Verification items for the finished model (mm, model axes). A direction names the side the tool comes from. Coordinates: 2 decimals unless noted, no trailing zeros. Write each loop counter-clockwise with the first axis right and the second up, starting at its lowest first coordinate (ties: lowest second). Pieces come first, ordered by that corner, then holes. Notation, with made-up numbers: (-36, 84) -> (17, 84) arc R12 cw to (17, 98) -> close; hole circle Ø1 at (84.5, -32.5). An arc over 180 degrees is marked (long way). Use CSV: the item, a comma, the result in double quotes.
```python
from build123d import *

# Parameters (mm, degrees)
CHAMFER1_SIZE  = 1
CHAMFER1_SIZE2 = 0.267949192


with BuildPart() as part:
    # Sketch1 → Revolve1 (revolve)
    with BuildSketch(Plane(origin=(0, 0, 0), x_dir=(1, 0, 0), z_dir=(0, 1, 0))):
        Polygon((16, 0), (16, 10), (15, 10), (15, 20), (45, 20), (45, 10), (21, 10), (21, 0), align=None)
    revolve(axis=Axis((0, 0, 0), (0, 0, 1)))

    # Chamfer1
    chamfer1_edges = [part.edges().sort_by_distance(p)[0] for p in [
        (-16, 0, 0),
    ]]
    chamfer1_side = [part.faces().sort_by_distance(p)[0] for p in [
        (-16, 0, -5),
    ]]
    chamfer(chamfer1_edges, length=CHAMFER1_SIZE, length2=CHAMFER1_SIZE2, reference=chamfer1_side[0])


solid = part.part
```
1) Cross-section at A-A (x = 0). Record the boundary of the cut face in (y, z).
Return value:
outline,"(-45, -20) -> (-15, -20) -> (-15, -10) -> (-16, -10) -> (-16, -1) -> (-16.27, 0) -> (-21, 0) -> (-21, -10) -> (-45, -10) -> close; (15, -20) -> (45, -20) -> (45, -10) -> (21, -10) -> (21, 0) -> (16.27, 0) -> (16, -1) -> (16, -10) -> (15, -10) -> close"
2) Mould release check, pull along X, two halves, no side actions. Record for faces 3 (the flat face through (6.1, -15.5, 0)), 4 (the cylindrical face through (20.765, -39.923, -14.93)), 5 (the cylindrical face through (-3.47, -15.62, -5.56)): released by +X, released by -X, zero draft, split by the parting line, or undercut.
Return value:
face 3,"zero draft"
face 4,"split by the parting line"
face 5,"undercut"
3) Cross-section at C-C (z = -15.75). Record the boundary of the cut face in (x, y), plus the area to 3 significant figures.
Return value:
outline,"circle Ø90 at (0, 0); hole circle Ø30 at (0, 0)"
area,"5,650 mm2"
4) Scan lines: L1, parallel to Y at x = 0, z = -17; L2, parallel to Z at x = 8.5, y = 27; L3, parallel to Y at x = 0, z = -3.5. Record each from-to range of solid material in increasing order.
Return value:
L1,"-45 to -15, 15 to 45"
L2,"-20 to -10"
L3,"-21 to -16, 16 to 21"
5) Cross-section at D-D (y = 37). Record the boundary of the cut face in (x, z), plus the area to 3 significant figures.
Return value:
outline,"(-25.61, -20) -> (25.61, -20) -> (25.61, -10) -> (-25.61, -10) -> close"
area,"512 mm2"
6) Set-up check for faces 1 (the cylindrical face through (-14.985, 0.66, -15.07)), 2 (the flat face through (9.4, -19.4, -10)): record each of +Z, -Z, +X, -X, +Y, -Y from which the full face is reachable in a straight line by a thin tool's end or side.
Return value:
face 1,"+Z, -Z"
face 2,"+Z"
7) Gauge pin test, flat ends, axial feed: pin 1 (1 mm diameter, centred on x = -0.5, z = -10, fed in from -Y); pin 2 (1.5 mm diameter, centred on y = 1, z = -14.5, fed in from -X); pin 3 (1 mm diameter, centred on x = 8, z = -11, fed in from +Y). Record the tip position at first contact, or that the pin passes through.
Return value:
pin 1,"y = -45"
pin 2,"x = -45"
pin 3,"y = 44.37"
